from build123d import *

# Parameters (mm, degrees)
PAD_DEPTH       = 19
SKETCH001_W     = 28.2
SKETCH001_H     = 24.2
POCKET_DEPTH    = 18.2
SKETCH002_W     = 23
SKETCH002_H     = 12
POCKET001_DEPTH = 0.8
SKETCH003_R     = 2
POCKET002_DEPTH = 1.4
SKETCH004_W     = 10
SKETCH004_H     = 3.5
POCKET003_DEPTH = 1.4
PAD001_DEPTH    = 2


with BuildPart() as part:
    # Sketch → Pad (new body)
    with BuildSketch(Plane.XY):
        with BuildLine():
            ThreePointArc((0, 2), (0.585786, 0.585786), (2, 0))
            Line((2, 0), (29, 0))
            ThreePointArc((29, 0), (30.414214, 0.585786), (31, 2))
            Line((31, 2), (31, 25))
            ThreePointArc((31, 25), (30.414214, 26.414214), (29, 27))
            Line((29, 27), (2, 27))
            ThreePointArc((2, 27), (0.585786, 26.414214), (0, 25))
            Line((0, 25), (0, 2))
        make_face()
    extrude(amount=PAD_DEPTH)

    # Sketch001 (on Face10 of Pad) → Pocket (cut)
    with BuildSketch(Plane.XY.offset(19)):
        with Locations((15.5, 13.5)):
            Rectangle(SKETCH001_W, SKETCH001_H)
    extrude(amount=-POCKET_DEPTH, mode=Mode.SUBTRACT)

    # Sketch002 (on Face15 of Pocket) → Pocket001 (cut)
    with BuildSketch(Plane.XY.offset(0.8)):
        with Locations((15.5, 18)):
            Rectangle(SKETCH002_W, SKETCH002_H)
    extrude(amount=-POCKET001_DEPTH, mode=Mode.SUBTRACT)

    # Sketch003 (on Face9 of Pocket001) → Pocket002 (cut)
    with BuildSketch(Plane.YZ.offset(31)):
        with Locations((11.5, 9)):
            Circle(SKETCH003_R)
        with Locations((17, 9)):
            Circle(SKETCH003_R)
        with Locations((22.5, 9)):
            Circle(SKETCH003_R)
    extrude(amount=-POCKET002_DEPTH, mode=Mode.SUBTRACT)

    # Sketch004 (on Face2 of Pocket002) → Pocket003 (cut)
    with BuildSketch(Plane(origin=(0, 0, 0), x_dir=(0, -1, 0), z_dir=(-1, 0, 0))):
        with Locations((-18, 5.05)):
            Rectangle(SKETCH004_W, SKETCH004_H)
    extrude(amount=-POCKET003_DEPTH, mode=Mode.SUBTRACT)

    # Sketch005 (on Face26 of Pocket003) → Pad001 (join)
    with BuildSketch(Plane.XY.offset(0.8)):
        Polygon((1.2, 25.6), (1.2, 4.9), (4, 4.9), (4, 5.9), (1.8, 5.9), (1.8, 25.6), align=None)
        Polygon((27, 4.9), (29.8, 4.9), (29.8, 25.6), (29.2, 25.6), (29.2, 5.9), (27, 5.9), align=None)
    extrude(amount=PAD001_DEPTH)


solid = part.part
Build history of the part. All positions in model axes, mm. A direction names the side the tool comes from. Round coordinates to 2 decimals unless told otherwise and drop trailing zeros. Loops run counter-clockwise (first coordinate to the right, second up) from the corner with the lowest first, then second, coordinate; pieces in that order, holes last. Notation, with made-up numbers: (21.25, 67.5) -> (60.25, 67.5) arc R16 cw to (60.25, 84.5) -> close; hole circle Ø11 at (-12.75, -23.75). An arc over 180 degrees is marked (long way). Answer in a Markdown table with one row per item.
Item 1: Drill centre lines: L1, parallel to Y at x = 17, z = 10.75; L2, parallel to X at y = 15, z = 10.75; L3, parallel to Z at x = 30.05, y = 11.5. Where is each one in solid material? Low to high. Write a range as [from, to].
Answers below:
| item | result |
|---|---|
| L1 | y = [0, 1.4], [25.6, 27] |
| L2 | x = [0, 1.4], [29.6, 31] |
| L3 | z = [0, 7], [11, 19] |
Item 2: Pin check, flat tips, straight feed: pin 1 (1.1 mm diameter, centred on x = 1, z = 5, fed in from +Y); pin 2 (1.1 mm diameter, centred on x = 1, y = 20.5, fed in from -Z); pin 3 (6 mm diameter, centred on x = 14, y = 6.5, fed in from +Z). Stop position of each tip, or through.
Answers below:
| item | result |
|---|---|
| pin 1 | stops at y = 26.95 |
| pin 2 | stops at z = 0 |
| pin 3 | stops at z = 0.8 |
Item 3: Saw through at D-D (z = 9). Write the cut outline in (x, y), and give its area (3 significant figures).
Answers below:
| item | result |
|---|---|
| outline | (0, 2) arc R2 ccw to (2, 0) -> (29, 0) arc R2 ccw to (31, 2) -> (31, 9.5) -> (29.6, 9.5) -> (29.6, 1.4) -> (1.4, 1.4) -> (1.4, 25.6) -> (29.6, 25.6) -> (29.6, 24.5) -> (31, 24.5) -> (31, 25) arc R2 ccw to (29, 27) -> (2, 27) arc R2 ccw to (0, 25) -> close; (29.6, 13.5) -> (31, 13.5) -> (31, 15) -> (29.6, 15) -> close; (29.6, 19) -> (31, 19) -> (31, 20.5) -> (29.6, 20.5) -> close |
| area | 134 mm² |
Item 4: Which spindle directions (+Z, -Z, +X, -X, +Y, -Y) get a long thin tool onto all of the face, cutting with end or side? Do faces 1 (the flat face through (1, 23, 5)), 2 (the cylindrical face through (30.43, 26.4, 9.37)), 3 (the flat face through (15, 25.6, 10)). Say none if no direction does.
Answers below:
| item | result |
|---|---|
| face 1 | -X |
| face 2 | +Z, -Z, +X, +Y |
| face 3 | +Z |
Item 5: Saw through at A-A (y = 11.5). Write the cut outline in (x, z).
Answers below:
| item | result |
|---|---|
| outline | (0, 0) -> (31, 0) -> (31, 7) -> (29.6, 7) -> (29.6, 2.8) -> (29.2, 2.8) -> (29.2, 0.8) -> (1.8, 0.8) -> (1.8, 2.8) -> (1.4, 2.8) -> (1.4, 19) -> (0, 19) -> close; (29.6, 11) -> (31, 11) -> (31, 19) -> (29.6, 19) -> close |
Item 6: Saw through at B-B (x = 17.5). Write the cut outline in (y, z), and give its area (3 significant figures).
Answers below:
| item | result |
|---|---|
| outline | (0, 0) -> (12, 0) -> (12, 0.8) -> (1.4, 0.8) -> (1.4, 19) -> (0, 19) -> close; (24, 0) -> (27, 0) -> (27, 19) -> (25.6, 19) -> (25.6, 0.8) -> (24, 0.8) -> close |
| area | 63.0 mm² |
Item 7: Mould opens along Y. For faces 4 (the flat face through (29.2, 16, 2)), 5 (the flat face through (15, 0, 9)), 6 (the flat face through (15, 1, 19)) say: +Y half, -Y half, draft (parallel to the pull), parting line (faces both ways), or undercut.
Answers below:
| item | result |
|---|---|
| face 4 | undercut |
| face 5 | -Y half |
| face 6 | draft |
Item 8: Saw through at C-C (y = 17). Write the cut outline in (x, z), and give its area (3 significant figures).
Answers below:
| item | result |
|---|---|
| outline | (0, 0) -> (4, 0) -> (4, 0.8) -> (1.8, 0.8) -> (1.8, 2.8) -> (1.4, 2.8) -> (1.4, 3.3) -> (0, 3.3) -> close; (0, 6.8) -> (1.4, 6.8) -> (1.4, 19) -> (0, 19) -> close; (27, 0) -> (31, 0) -> (31, 7) -> (29.6, 7) -> (29.6, 2.8) -> (29.2, 2.8) -> (29.2, 0.8) -> (27, 0.8) -> close; (29.6, 11) -> (31, 11) -> (31, 19) -> (29.6, 19) -> close |
| area | 48.5 mm² |
